from build123d import *

# Parameters (mm, degrees)
SKETCH2_W           = 131.4
SKETCH2_H           = 62.2
BOSS_EXTRUDE1_DEPTH = 14.7
SKETCH3_W           = 127.6
SKETCH3_H           = 58.4
CUT_EXTRUDE1_DEPTH  = 13
SKETCH4_W           = 20.3
SKETCH4_H           = 9.9
BOSS_EXTRUDE2_DEPTH = 2.2
FILLET1_R           = 3


with BuildPart() as part:
    # Sketch2 → Boss-Extrude1 (new body)
    with BuildSketch(Plane(origin=(0, 0, 0), x_dir=(1, 0, 0), z_dir=(0, 1, 0))):
        Rectangle(SKETCH2_W, SKETCH2_H)
    extrude(amount=BOSS_EXTRUDE1_DEPTH)

    # Sketch3 → Cut-Extrude1 (cut)
    with BuildSketch(Plane(origin=(0, 14.7, 0), x_dir=(1, 0, 0), z_dir=(0, 1, 0))):
        Rectangle(SKETCH3_W, SKETCH3_H)
    extrude(amount=-CUT_EXTRUDE1_DEPTH, mode=Mode.SUBTRACT)

    # Sketch4 → Boss-Extrude2 (add)
    with BuildSketch(Plane.XZ):
        with Locations((0, 36.05)):
            Rectangle(SKETCH4_W, SKETCH4_H)
    extrude(amount=-BOSS_EXTRUDE2_DEPTH)

    # Fillet1
    fillet1_edges = [part.edges().sort_by_distance(p)[0] for p in [
        (-10.15, 1.1, 41),
        (10.15, 1.1, 41),
    ]]
    fillet(fillet1_edges, radius=FILLET1_R)


solid = part.part
Design review of the part built by this model. Coordinates are the model's own, in mm. A direction names the side the tool comes from. Round coordinates to 2 decimals unless told otherwise and drop trailing zeros. Write each loop counter-clockwise with the first axis right and the second up, starting at its lowest first coordinate (ties: lowest second). Pieces come first, ordered by that corner, then holes.
Item 1: Consider section C-C on z = -2.5. Give the boundary of the cut face in (x, y).
Item 2: For faces 1 (the flat face through (0, 2.2, 36)), 2 (the flat face through (-1, 8, -29.2)), 3 (the flat face through (0, 14.7, -30)), list the 3-axis set-ups (+Z, -Z, +X, -X, +Y, -Y) from which the entire face can be reached by the end or side of a thin tool; tool diameter is ignored.
Item 3: For pin 1 Ø6.5 at (x, y) = (4, 10.5) entering from +Z; pin 2 Ø1.5 at (x, z) = (-4, -23.5) entering from +Y; pin 3 Ø1.8 at (y, z) = (0.5, 33) entering from +X, all flat-tipped, find the tip position at first contact; note any pin that passes through.
Item 4: Draft analysis for pull direction Z (two halves, no side actions). For faces 4 (the flat face through (-1, 0, 4)), 5 (the flat face through (-63.8, 8, 0)), 6 (the cylindrical face through (9.29, 1.12, 40.1)), state which applies: released by +Z, released by -Z, zero draft, split by the parting line, or undercut.
Item 5: Wall thickness on L1, parallel to X at y = 8.25, z = 17; L2, parallel to Z at x = -7, y = 9.75; L3, parallel to Y at x = 41, z = -18: over which ranges is each line inside the solid? List them lowest first.
Item 6: Consider section B-B on x = -17. Give the boundary of the cut face in (y, z).
Item 7: Consider section A-A on y = 13. Give the boundary of the cut face in (x, z), and give its area (3 significant figures).
Check values:
1. outline: (-65.7, 0) - (65.7, 0) - (65.7, 14.7) - (63.8, 14.7) - (63.8, 1.7) - (-63.8, 1.7) - (-63.8, 14.7) - (-65.7, 14.7) - close
2. face 1: +Z, +X, -X, +Y
2. face 2: +Y
2. face 3: +Z, -Z, +X, -X, +Y
3. pin 1: stops at z = 31.1
3. pin 2: stops at y = 1.7
3. pin 3: stops at x = 10.15
4. face 4: zero draft
4. face 5: undercut
4. face 6: released by +Z
5. L1: x = -65.7 to -63.8, 63.8 to 65.7
5. L2: z = -31.1 to -29.2, 29.2 to 31.1
5. L3: y = 0 to 1.7
6. outline: (0, -31.1) - (14.7, -31.1) - (14.7, -29.2) - (1.7, -29.2) - (1.7, 29.2) - (14.7, 29.2) - (14.7, 31.1) - (0, 31.1) - close
7. outline: (-65.7, -31.1) - (65.7, -31.1) - (65.7, 31.1) - (-65.7, 31.1) - close; hole (-63.8, -29.2) - (63.8, -29.2) - (63.8, 29.2) - (-63.8, 29.2) - close
7. area: 721 mm2
